CAD build for the part. Positions are in the model's coordinates, mm. Face numbers are marked on the shaded views. A direction names the side the tool comes from. Coordinates: 2 decimals unless noted, no trailing zeros. Write each loop counter-clockwise with the first axis right and the second up, starting at its lowest first coordinate (ties: lowest second). Pieces come first, ordered by that corner, then holes. Notation, with made-up numbers: (21, 11) - (55, 11) arc R12 ccw to (55, 19) - close; hole circle Ø6 at (23, 79). An arc over 180 degrees is marked (long way). One line per question, with ' | ' between items. Start each with the question number.
1. Flat gauge pins, fed straight in: P1, Ø3.5, axis at x = 15, z = 0, coming from the +Y side; P2, Ø1, axis at x = 8.5, y = 6, coming from the +Z side; P3, Ø3, axis at y = 4, z = -2, coming from the +X side; P4, Ø2, axis at x = 21, y = 4, coming from the -Z side. Where does each tip first touch, or does it go through?
2. Two-plate mould, pull along X, no slides. Class the marked faces 6, 7, 8 and 9: +X half, -X half, draft (parallel to the pull), parting line (faces both ways), or undercut.
3. Band-saw the part on C-C, the plane x = 15. Write the cut outline in (y, z).
4. Which spindle directions (+Z, -Z, +X, -X, +Y, -Y) get a long thin tool onto all of the face, cutting with end or side? Do the marked faces 1, 2, 3, 4 and 5. Say none if no direction does.
5. Band-saw the part on D-D, the plane y = 1.25. Write the cut outline in (x, z), then the cut area to 3 significant figures.
6. Probe line 1 (X direction, y = 1, z = -2); line 2 (Z direction, x = 30, y = 8.85); line 3 (X direction, y = 8.75, z = -2.25). List the from-to ranges inside material, lowest first.
7. Band-saw the part on A-A, the plane z = 0. Write the cut outline in (x, y).
8. Band-saw the part on B-B, the plane y = 5. Write the cut outline in (x, z), then the cut area to 3 significant figures.
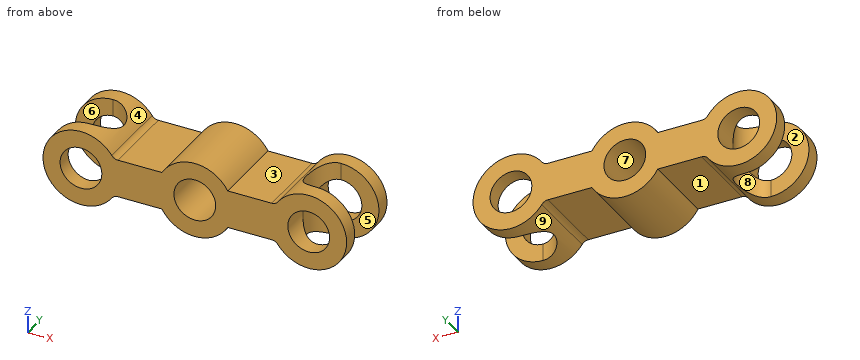
from build123d import *

# Parameters (mm, degrees)
SKETCH1_W            = 15
SKETCH1_H            = 5
BOSS_EXTRUDE1_DEPTH  = 10
SKETCH2_R            = 5
BOSS_EXTRUDE2_DEPTH  = 10
CUT_EXTRUDE1_REACH   = 20.708
SKETCH3_R            = 2.75
CUT_EXTRUDE2_DEPTH   = 19.708286934
FILLET1_R            = 1
FILLET1_OF_MIRROR1_R = 1
SKETCH6_R            = 5
BOSS_EXTRUDE3_DEPTH  = 10
SKETCH7_R            = 2.75
CUT_EXTRUDE3_DEPTH   = 10


with BuildPart() as part:
    # Sketch1 → Boss-Extrude1 (new body)
    with BuildSketch(Plane(origin=(0, 0, 0), x_dir=(1, 0, 0), z_dir=(0, 1, 0))):
        with Locations((7.5, 0)):
            Rectangle(SKETCH1_W, SKETCH1_H)
    boss_extrude1 = extrude(amount=BOSS_EXTRUDE1_DEPTH)

    # Sketch2 → Boss-Extrude2 (add)
    with BuildSketch(Plane(origin=(0, 0, 0), x_dir=(1, 0, 0), z_dir=(0, 1, 0))):
        Circle(SKETCH2_R)
    boss_extrude2 = extrude(amount=BOSS_EXTRUDE2_DEPTH)

    # Sketch3 → Cut-Extrude1 (cut, up to next)
    with BuildSketch(Plane(origin=(0, 0, 0), x_dir=(1, 0, 0), z_dir=(0, 1, 0)), mode=Mode.PRIVATE) as cut_extrude1_sk1:
        with Locations(Location((0, 0, 0), (0, 0, 270))):
            Circle(SKETCH3_R)
    cut_extrude1_tool1 = extrude(cut_extrude1_sk1.sketch, amount=CUT_EXTRUDE1_REACH, mode=Mode.PRIVATE) & part.part
    cut_extrude1 = cut_extrude1_tool1.solids().sort_by_distance((0, 0, 0))[0]
    add(cut_extrude1, mode=Mode.SUBTRACT)

    # Sketch4 → Cut-Extrude2 (cut, symmetric)
    with BuildSketch(Plane.XY):
        with BuildLine():
            Line((0, 8), (-5, 8))
            Line((-5, 8), (-5, 2))
            Line((-5, 2), (0, 2))
            ThreePointArc((0, 2), (3, 5), (0, 8))
        make_face()
    cut_extrude2 = extrude(amount=CUT_EXTRUDE2_DEPTH, both=True, mode=Mode.SUBTRACT)

    # Fillet1
    fillet1_edges = [part.edges().sort_by_distance(p)[0] for p in [
        (4.330127019, 5, 2.5),
        (4.330127019, 5, -2.5),
    ]]
    fillet(fillet1_edges, radius=FILLET1_R)

    # Mirror1: Boss-Extrude1, Boss-Extrude2, Cut-Extrude1, Cut-Extrude2 across plane
    add(boss_extrude1.mirror(Plane(origin=(15, 10, -2.5), x_dir=(0, 0, 1), z_dir=(-1, 0, 0))))
    add(boss_extrude2.mirror(Plane(origin=(15, 10, -2.5), x_dir=(0, 0, 1), z_dir=(-1, 0, 0))))
    add(cut_extrude1.mirror(Plane(origin=(15, 10, -2.5), x_dir=(0, 0, 1), z_dir=(-1, 0, 0))), mode=Mode.SUBTRACT)
    add(cut_extrude2.mirror(Plane(origin=(15, 10, -2.5), x_dir=(0, 0, 1), z_dir=(-1, 0, 0))), mode=Mode.SUBTRACT)

    # Fillet1 of Mirror1
    fillet1_of_mirror1_edges = [part.edges().sort_by_distance(p)[0] for p in [
        (25.669872981, 5, 2.5),
        (25.669872981, 5, -2.5),
    ]]
    fillet(fillet1_of_mirror1_edges, radius=FILLET1_OF_MIRROR1_R)

    # Sketch6 → Boss-Extrude3 (add)
    with BuildSketch(Plane(origin=(0, 0, 0), x_dir=(1, 0, 0), z_dir=(0, 1, 0))):
        with Locations((15, 0)):
            Circle(SKETCH6_R)
    extrude(amount=BOSS_EXTRUDE3_DEPTH)

    # Sketch7 → Cut-Extrude3 (cut)
    with BuildSketch(Plane(origin=(0, 0, 0), x_dir=(1, 0, 0), z_dir=(0, 1, 0))):
        with Locations(Location((15, 0, 0), (0, 0, 270))):
            Circle(SKETCH7_R)
    extrude(amount=CUT_EXTRUDE3_DEPTH, mode=Mode.SUBTRACT)


solid = part.part
Filled in:
1) P1: passes through | P2: stops at z = 2.5 | P3: stops at x = 28.33 | P4: stops at z = -2.5
2) face 6: draft | face 7: undercut | face 8: -X half | face 9: undercut
3) outline: (0, -5) - (10, -5) - (10, -2.75) - (0, -2.75) - close; (0, 2.75) - (10, 2.75) - (10, 5) - (0, 5) - close
4) face 1: -Z, +Y, -Y | face 2: +Z, -Z, -X | face 3: +Z, +Y, -Y | face 4: +Y, -Y | face 5: +Z, -Z, +X
5) outline: (4.06, -2.92) arc R1 cw to (4.87, -2.5) - (10.67, -2.5) arc R5 ccw to (19.33, -2.5) - (25.13, -2.5) arc R1 cw to (25.94, -2.92) arc R5 ccw (long way) to (25.94, 2.92) arc R1 cw to (25.13, 2.5) - (19.33, 2.5) arc R5 ccw to (10.67, 2.5) - (4.87, 2.5) arc R1 cw to (4.06, 2.92) arc R5 ccw (long way) to start; hole circle Ø5.5 at (0, 0); hole circle Ø5.5 at (15, 0); hole circle Ø5.5 at (30, 0) | area: 219 mm²
6) line 1: x = -4.58 to -1.89, 1.89 to 13.11, 16.89 to 28.11, 31.89 to 34.58 | line 2: z = -5 to -2.75, 2.75 to 5 | line 3: x = -4.47 to -1.58, 1.58 to 13.42, 16.58 to 28.42, 31.58 to 34.47
7) outline: (-5, 0) - (-2.75, 0) - (-2.75, 2) - (-5, 2) - close; (-5, 8) - (-2.75, 8) - (-2.75, 10) - (-5, 10) - close; (2.75, 0) - (12.25, 0) - (12.25, 10) - (2.75, 10) - (2.75, 6.2) arc R3 cw to (2.75, 3.8) - close; (17.75, 0) - (27.25, 0) - (27.25, 3.8) arc R3 cw to (27.25, 6.2) - (27.25, 10) - (17.75, 10) - close; (32.75, 0) - (35, 0) - (35, 2) - (32.75, 2) - close; (32.75, 8) - (35, 8) - (35, 10) - (32.75, 10) - close
8) outline: (3, -4) arc R5 ccw to (4.06, -2.92) arc R1 cw to (4.87, -2.5) - (10.67, -2.5) arc R5 ccw to (19.33, -2.5) - (25.13, -2.5) arc R1 cw to (25.94, -2.92) arc R5 ccw to (27, -4) - (27, 4) arc R5 ccw to (25.94, 2.92) arc R1 cw to (25.13, 2.5) - (19.33, 2.5) arc R5 ccw to (10.67, 2.5) - (4.87, 2.5) arc R1 cw to (4.06, 2.92) arc R5 ccw to (3, 4) - close; hole circle Ø5.5 at (15, 0) | area: 132 mm²
